```python
from build123d import *

# Parameters (mm, degrees)
SKETCH1_W                = 8.7
SKETCH1_H                = 4.35
BOSS_EXTRUDE1_DEPTH      = 4.68
SKETCH3_W                = 2
SKETCH3_H                = 2
BOSS_EXTRUDE3_DEPTH      = 4
SKETCH4_W                = 0.42
SKETCH4_H                = 1.17
SKETCH4_W_2              = 0.5
SKETCH4_H_2              = 0.3
BOSS_EXTRUDE4_DEPTH      = 2.75
CHAMFER1_SIZE            = 0.5
CHAMFER1_OF_MIRROR1_SIZE = 0.5


with BuildPart() as part:
    # Sketch1 → Boss-Extrude1 (new body)
    with BuildSketch(Plane(origin=(0, 0, 0), x_dir=(1, 0, 0), z_dir=(0, 1, 0))):
        Rectangle(SKETCH1_W, SKETCH1_H)
    extrude(amount=BOSS_EXTRUDE1_DEPTH)

    # Sketch3 → Boss-Extrude3 (add)
    with BuildSketch(Plane(origin=(0, 0, -2.175), x_dir=(-1, 0, 0), z_dir=(0, 0, -1))):
        with Locations((-0.85, 2.34)):
            Rectangle(SKETCH3_W, SKETCH3_H)
    extrude(amount=BOSS_EXTRUDE3_DEPTH)

    # Sketch4 → Boss-Extrude4 (add)
    with BuildSketch(Plane.XZ):
        with Locations((4.14, 0)):
            Rectangle(SKETCH4_W, SKETCH4_H)
        with Locations((1.93, 0)):
            Rectangle(SKETCH4_W_2, SKETCH4_H_2)
    boss_extrude4 = extrude(amount=BOSS_EXTRUDE4_DEPTH)

    # Chamfer1
    chamfer1_edges = [part.edges().sort_by_distance(p)[0] for p in [
        (4.14, -2.75, 0.585),
        (4.14, -2.75, -0.585),
    ]]
    chamfer(chamfer1_edges, length=CHAMFER1_SIZE)

    # Mirror1: Boss-Extrude4 across plane
    add(boss_extrude4.mirror(Plane(origin=(0, 0, 0), x_dir=(0, 0, 1), z_dir=(1, 0, 0))))

    # Chamfer1 of Mirror1
    chamfer1_of_mirror1_edges = [part.edges().sort_by_distance(p)[0] for p in [
        (-4.14, -2.75, 0.585),
        (-4.14, -2.75, -0.585),
    ]]
    chamfer(chamfer1_of_mirror1_edges, length=CHAMFER1_OF_MIRROR1_SIZE)


solid = part.part
```
Design review of the part built by this model. Coordinates are the model's own, in mm. A direction names the side the tool comes from. Coordinates: 2 decimals unless noted, no trailing zeros. Order: outer loops, then holes, each group sorted by start corner. A loop starts at its lowest first (then second) coordinate and runs counter-clockwise, first axis right, second up. Notation, with made-up numbers: (10, -33.75) - (20, -33.75) arc R32 cw to (20, -6.75) - close; hole circle Ø8 at (-17.5, -24). An arc over 180 degrees is marked (long way). One line per question, with ' | ' between items.
Q1. For faces 1 (the flat face through (1.85, 2, -4)), 2 (the flat face through (1, 3.34, -4)), 3 (the flat face through (1, 1.34, -4)), 4 (the flat face through (-0.15, 2, -4)), 5 (the flat face through (-3.93, -1, 0)), list the 3-axis set-ups (+Z, -Z, +X, -X, +Y, -Y) from which the entire face can be reached by the end or side of a thin tool; tool diameter is ignored.
Answer key:
face 1: -Z, +X, +Y, -Y | face 2: -Z, +X, -X, +Y | face 3: -Z, +X, -X, -Y | face 4: -Z, -X, +Y, -Y | face 5: +Z, -Z, -Y
Q2. To check wall thickness, follow line 1 along Y through (x, z) = (3.5, 0.25); line 2 along X through (y, z) = (2.25, -2.75); line 3 along Z through (x, y) = (-0.75, 3.5) (3 decimals). State the ranges of each line that lie inside material, in increasing order.
Answer key:
line 1: y = 0 to 4.68 | line 2: x = -0.15 to 1.85 | line 3: z = -2.175 to 2.175
Q3. Consider section B-B, the plane x = 0.5. Give the boundary of the cut face in (y, z) (3 decimals).
Answer key:
outline: (0, -2.175) - (1.34, -2.175) - (1.34, -6.175) - (3.34, -6.175) - (3.34, -2.175) - (4.68, -2.175) - (4.68, 2.175) - (0, 2.175) - close
Q4. The part is to be moulded in two halves that separate along X. For faces 6 (the flat face through (4.35, 2, 0)), 7 (the flat face through (-4.35, 2, 0)), 8 (the flat face through (3.93, -1, 0)), say which applies: +X half, -X half, draft (parallel to the pull), parting line (faces both ways), or undercut.
Answer key:
face 6: +X half | face 7: -X half | face 8: undercut
Q5. Clearance check with flat-ended pins moving along their axes: pin 1 Ø0.6 at (y, z) = (2, -4) entering from +X; pin 2 Ø1 at (y, z) = (-0.5, -4.5) entering from +X (3 decimals); pin 3 Ø1 at (x, z) = (0.5, -5) entering from +Y; pin 4 Ø1 at (y, z) = (2.5, -3.5) entering from -X. State where each tip first meets the part, or that it passes through.
Answer key:
pin 1: stops at x = 1.85 | pin 2: passes through | pin 3: stops at y = 3.34 | pin 4: stops at x = -0.15
Q6. Consider section C-C, the plane y = 2.5. Give the boundary of the cut face in (x, z) (3 decimals).
Answer key:
outline: (-4.35, -2.175) - (-0.15, -2.175) - (-0.15, -6.175) - (1.85, -6.175) - (1.85, -2.175) - (4.35, -2.175) - (4.35, 2.175) - (-4.35, 2.175) - close
Q7. Consider section D-D, the plane z = -3. Give the boundary of the cut face in (x, y), then the cut area to 3 significant figures.
Answer key:
outline: (-0.15, 1.34) - (1.85, 1.34) - (1.85, 3.34) - (-0.15, 3.34) - close | area: 4.00 mm2
Q8. Consider section A-A, the plane y = -1.25. Give the boundary of the cut face in (x, z) (3 decimals).
Answer key:
outline: (-4.35, -0.585) - (-3.93, -0.585) - (-3.93, 0.585) - (-4.35, 0.585) - close; (-2.18, -0.15) - (-1.68, -0.15) - (-1.68, 0.15) - (-2.18, 0.15) - close; (1.68, -0.15) - (2.18, -0.15) - (2.18, 0.15) - (1.68, 0.15) - close; (3.93, -0.585) - (4.35, -0.585) - (4.35, 0.585) - (3.93, 0.585) - close
